```python
from build123d import *

# Parameters (mm, degrees)
SKETCH1_W           = 22.225
SKETCH1_H           = 50.8
BOSS_EXTRUDE1_DEPTH = 38.1
FILLET1_R           = 25.4
SKETCH2_R           = 7.9375
CUT_EXTRUDE1_DEPTH  = 38.1


with BuildPart() as part:
    # Sketch1 → Boss-Extrude1 (new body)
    with BuildSketch(Plane.XY):
        with Locations((11.1125, 25.4)):
            Rectangle(SKETCH1_W, SKETCH1_H)
    extrude(amount=BOSS_EXTRUDE1_DEPTH)

    # Fillet1
    fillet1_edges = [part.edges().sort_by_distance(p)[0] for p in [
        (11.1125, 0, 38.1),
        (11.1125, 50.8, 38.1),
    ]]
    fillet(fillet1_edges, radius=FILLET1_R - 0.0001)  # a hair under: the kernel refuses the full size

    # Sketch2 → Cut-Extrude1 (cut)
    with BuildSketch(Plane(origin=(22.225, 0, 0), x_dir=(0, 0, -1), z_dir=(1, 0, 0))):
        with Locations(Location((-19.05, 25.4, 0), (0, 0, 90))):
            Circle(SKETCH2_R)
    extrude(amount=-CUT_EXTRUDE1_DEPTH, mode=Mode.SUBTRACT)


solid = part.part
```
Here's how the part is built. I have some questions about the finished solid (model axes, mm). Give positions to 0.01 mm unless a question says otherwise; leave off trailing zeros. Write each loop counter-clockwise with the first axis right and the second up, starting at its lowest first coordinate (ties: lowest second). Pieces come first, ordered by that corner, then holes. Notation, with made-up numbers: (21.5, -33.5) -> (54.5, -33.5) arc R25 cw to (54.5, -15.5) -> close; hole circle Ø9 at (34, 72.25). An arc over 180 degrees is marked (long way). Write each question's results on one line, items separated by ' | '.
Item 1: Suppose I cut it at B-B on z = 19.05. Write out the boundary of the cut face in (x, y) (1 decimal).
Output:
outline: (0, 0.8) -> (22.2, 0.8) -> (22.2, 17.5) -> (0, 17.5) -> close; (0, 33.3) -> (22.2, 33.3) -> (22.2, 50) -> (0, 50) -> close
Item 2: For pin 1 Ø3 at (y, z) = (10, 21.5) entering from -X; pin 2 Ø1.5 at (x, z) = (7.5, 16.5) entering from -Y; pin 3 Ø5 at (x, y) = (16.5, 22.5) entering from +Z; pin 4 Ø4 at (x, y) = (4, 41) entering from +Z, each with a flat end and sliding along its axis, tell me the tip position at first contact or that it passes through.
Output:
pin 1: stops at x = 0 | pin 2: stops at y = 0.18 | pin 3: stops at z = 38.1 | pin 4: stops at z = 34.15
Item 3: Suppose I cut it at D-D on z = 29. Write out the boundary of the cut face in (x, y) (3 decimals), plus the area to 3 significant figures.
Output:
outline: (0, 5.92) -> (22.225, 5.92) -> (22.225, 44.88) -> (0, 44.88) -> close | area: 866 mm^2
Item 4: If I drill on L1, parallel to Z at x = 13, y = 25.5; L2, parallel to Y at x = 4.5, z = 13; L3, parallel to Y at x = 18.5, z = 22.5, over which ranges is the centre line in solid material (lowest first)?
Output:
L1: z = 0 to 11.11, 26.99 to 38.1 | L2: y = 0 to 20.26, 30.54 to 50.8 | L3: y = 1.97 to 18.25, 32.55 to 48.83
Item 5: Suppose I cut it at C-C on y = 7. Write out the boundary of the cut face in (x, z) (3 decimals).
Output:
outline: (0, 0) -> (22.225, 0) -> (22.225, 30.21) -> (0, 30.21) -> close
Item 6: We'd pull the mould along Y, two halves only. Please class faces 1 (the face through (11, 50.8, 6)), 2 (the face through (11, 26, 0)), 3 (the face through (11.27, 7.24, 30.46)), 4 (the face through (11.27, 17.47, 19.4)): pulls with the +Y half, pulls with the -Y half, needs draft (parallel to the pull), parting line crosses it, or undercut.
Output:
face 1: pulls with the +Y half | face 2: needs draft | face 3: pulls with the -Y half | face 4: undercut
